Work out the finished part from the listing and answer in its coordinate system (mm). A direction names the side the tool comes from. Give positions to 0.01 mm unless a question says otherwise; leave off trailing zeros. Write each loop counter-clockwise with the first axis right and the second up, starting at its lowest first coordinate (ties: lowest second). Pieces come first, ordered by that corner, then holes. Notation, with made-up numbers: (86, 75.5) - (121, 75.5) arc R17 ccw to (121, 97.5) - close; hole circle Ø7 at (84, 85.25). An arc over 180 degrees is marked (long way). Write item = value, one per line.
from build123d import *

# Parameters (mm, degrees)
SKETCH1_R           = 10.5791
BOSS_EXTRUDE1_DEPTH = 16.256
SKETCH2_R           = 7.874
CUT_EXTRUDE1_DEPTH  = 13.97
FILLET1_R           = 1.27
FILLET2_R           = 2.54
SKETCH4_R           = 1.143
CUT_EXTRUDE2_DEPTH  = 21.469382398


with BuildPart() as part:
    # Sketch1 → Boss-Extrude1 (new body)
    with BuildSketch(Plane(origin=(0, 0, 0), x_dir=(1, 0, 0), z_dir=(0, 1, 0))):
        with Locations(Location((0, 0, 0), (0, 0, 270))):
            Circle(SKETCH1_R)
    extrude(amount=BOSS_EXTRUDE1_DEPTH)

    # Sketch2 → Cut-Extrude1 (cut)
    with BuildSketch(Plane(origin=(0, 16.256, 0), x_dir=(1, 0, 0), z_dir=(0, 1, 0))):
        with Locations(Location((0, 0, 0), (0, 0, 270))):
            Circle(SKETCH2_R)
    extrude(amount=-CUT_EXTRUDE1_DEPTH, mode=Mode.SUBTRACT)

    # Fillet1
    fillet1_edges = [part.edges().sort_by_distance(p)[0] for p in [
        (0, 16.256, -10.5791),
    ]]
    fillet(fillet1_edges, radius=FILLET1_R)

    # Fillet2
    fillet2_edges = [part.edges().sort_by_distance(p)[0] for p in [
        (0, 0, -10.5791),
    ]]
    fillet(fillet2_edges, radius=FILLET2_R)

    # Sketch4 → Cut-Extrude2 (cut, through all)
    with BuildSketch(Plane(origin=(0, 2.286, 0), x_dir=(1, 0, 0), z_dir=(0, 1, 0))):
        with Locations(Location((0, 0, 0), (0, 0, 270))):
            Circle(SKETCH4_R)
    extrude(amount=-CUT_EXTRUDE2_DEPTH, mode=Mode.SUBTRACT)


solid = part.part
1. For a pull along X with two mould halves and no side action, classify faces 1 (the flat face through (2, 16.256, -8)), 2 (the cylindrical face through (-7.687, 9.369, -1.707)), 3 (the cylindrical face through (8.92, 8.68, 5.69)) as pulls with the +X half, pulls with the -X half, needs draft (parallel to the pull), parting line crosses it, or undercut.
Solution:
face_1 = needs draft
face_2 = undercut
face_3 = parting line crosses it
2. A tool of negligible diameter and unlimited length cuts with its end or side. For faces 4 (the cylindrical face through (-1.014, 1.159, 0.527)), 5 (the flat face through (-2, 2.286, 0)), from which of +Z, -Z, +X, -X, +Y, -Y can it reach the whole face along a straight path? Write none if from no direction.
Solution:
face_4 = +Y, -Y
face_5 = +Y
3. Find section A-A, the plane x = 0. Give the vertices of the cut face in (y, z), then the cut area to 3 significant figures.
Solution:
outline = (0, -8.04) arc R2.54 ccw to (2.54, -10.58) - (14.99, -10.58) arc R1.27 ccw to (16.26, -9.31) - (16.26, -7.87) - (2.29, -7.87) - (2.29, -1.14) - (0, -1.14) - close; (0, 1.14) - (2.29, 1.14) - (2.29, 7.87) - (16.26, 7.87) - (16.26, 9.31) arc R1.27 ccw to (14.99, 10.58) - (2.54, 10.58) arc R2.54 ccw to (0, 8.04) - close
area = 115 mm^2
4. Find section C-C, the plane y = 4.5. Give the vertices of the cut face in (x, z), then the cut area to 3 significant figures.
Solution:
outline = circle Ø21.16 at (0, 0); hole circle Ø15.75 at (0, 0)
area = 157 mm^2
5. Find section B-B, the plane z = 0. Give the vertices of the cut face in (x, y), then the cut area to 3 significant figures.
Solution:
outline = (-10.58, 2.54) arc R2.54 ccw to (-8.04, 0) - (-1.14, 0) - (-1.14, 2.29) - (-7.87, 2.29) - (-7.87, 16.26) - (-9.31, 16.26) arc R1.27 ccw to (-10.58, 14.99) - close; (1.14, 0) - (8.04, 0) arc R2.54 ccw to (10.58, 2.54) - (10.58, 14.99) arc R1.27 ccw to (9.31, 16.26) - (7.87, 16.26) - (7.87, 2.29) - (1.14, 2.29) - close
area = 115 mm^2
6. Find section D-D, the plane y = 1. Give the vertices of the cut face in (x, z).
Solution:
outline = circle Ø20.12 at (0, 0); hole circle Ø2.29 at (0, 0)
7. Straight lines are drawn through the part: line 1 (X direction, y = 11.75, z = 0); line 2 (Y direction, x = 1.5, z = 5.5); line 3 (X direction, y = 5.75, z = -7). For each, find the intervals that lie inside material, in ascending order.
Solution:
line_1 = -10.58 to -7.87, 7.87 to 10.58
line_2 = 0 to 2.29
line_3 = -7.93 to -3.61, 3.61 to 7.93
8. Given pin 1 (4 mm diameter, centred on x = 3.5, y = 4, fed in from -Z); pin 2 (1 mm diameter, centred on y = 8, z = -8.5, fed in from -X); pin 3 (6 mm diameter, centred on x = -5.5, y = 13.5, fed in from -Z); pin 4 (12 mm diameter, centred on x = -5.5, z = 2.5, fed in from -Y), each flat-ended and moving along its own axis, determine where each tip first touches the part or whether it passes through.
Solution:
pin_1 = -10.47
pin_2 = -6.92
pin_3 = -10.28
pin_4 = 0
